from build123d import *

# Parameters (mm, degrees)
SKETCH2_W           = 15
SKETCH2_H           = 20
SKETCH2_W_2         = 23
SKETCH2_H_2         = 15
BOSS_EXTRUDE1_DEPTH = 10


with BuildPart() as part:
    # Sketch2 → Boss-Extrude1 (new body)
    with BuildSketch(Plane.XY):
        Polygon((0, 0), (120, 0), (120, 10), (180, 10), (180, 0), (240, 0), (240, 10), (300, 10), (300, 0), (420, 0), (420, -75), (430, -75), (430, -120), (420, -120), (420, -165), (430, -165), (430, -210), (420, -210), (420, -285), (300, -285), (300, -295), (240, -295), (240, -285), (180, -285), (180, -295), (120, -295), (120, -285), (0, -285), (0, -210), (-10, -210), (-10, -165), (0, -165), (0, -120), (-10, -120), (-10, -75), (0, -75), align=None)
        with Locations((144.916665259, -151.561421388)):
            Rectangle(SKETCH2_W, SKETCH2_H, mode=Mode.SUBTRACT)
        with Locations((338.315226992, -153.118682745)):
            Rectangle(SKETCH2_W, SKETCH2_H, mode=Mode.SUBTRACT)
        with Locations((376.315226992, -153.118682745)):
            Rectangle(SKETCH2_W, SKETCH2_H, mode=Mode.SUBTRACT)
        with Locations((338.315226992, -239.118682745)):
            Rectangle(SKETCH2_W, SKETCH2_H, mode=Mode.SUBTRACT)
        with Locations((44.5, -152)):
            Rectangle(SKETCH2_W, SKETCH2_H, mode=Mode.SUBTRACT)
        with Locations((82.5, -152)):
            Rectangle(SKETCH2_W, SKETCH2_H, mode=Mode.SUBTRACT)
        with Locations((44.5, -238)):
            Rectangle(SKETCH2_W, SKETCH2_H, mode=Mode.SUBTRACT)
        with Locations((82.5, -238)):
            Rectangle(SKETCH2_W, SKETCH2_H, mode=Mode.SUBTRACT)
        with Locations((63.5, -193.5)):
            Rectangle(SKETCH2_W_2, SKETCH2_H_2, mode=Mode.SUBTRACT)
        with Locations((182.916665259, -151.561421388)):
            Rectangle(SKETCH2_W, SKETCH2_H, mode=Mode.SUBTRACT)
        with Locations((144.916665259, -237.561421388)):
            Rectangle(SKETCH2_W, SKETCH2_H, mode=Mode.SUBTRACT)
        with Locations((182.916665259, -237.561421388)):
            Rectangle(SKETCH2_W, SKETCH2_H, mode=Mode.SUBTRACT)
        with Locations((163.916665259, -193.061421388)):
            Rectangle(SKETCH2_W_2, SKETCH2_H_2, mode=Mode.SUBTRACT)
        with Locations((242.869049507, -152.216184795)):
            Rectangle(SKETCH2_W, SKETCH2_H, mode=Mode.SUBTRACT)
        with Locations((280.869049507, -152.216184795)):
            Rectangle(SKETCH2_W, SKETCH2_H, mode=Mode.SUBTRACT)
        with Locations((242.869049507, -238.216184795)):
            Rectangle(SKETCH2_W, SKETCH2_H, mode=Mode.SUBTRACT)
        with Locations((280.869049507, -238.216184795)):
            Rectangle(SKETCH2_W, SKETCH2_H, mode=Mode.SUBTRACT)
        with Locations((261.869049507, -193.716184795)):
            Rectangle(SKETCH2_W_2, SKETCH2_H_2, mode=Mode.SUBTRACT)
        with Locations((376.315226992, -239.118682745)):
            Rectangle(SKETCH2_W, SKETCH2_H, mode=Mode.SUBTRACT)
        with Locations((357.315226992, -194.618682745)):
            Rectangle(SKETCH2_W_2, SKETCH2_H_2, mode=Mode.SUBTRACT)
    extrude(amount=BOSS_EXTRUDE1_DEPTH)


solid = part.part
Verification items for the finished model (mm, model axes). A direction names the side the tool comes from. Give positions to 0.01 mm unless a question says otherwise; leave off trailing zeros. Write each loop counter-clockwise with the first axis right and the second up, starting at its lowest first coordinate (ties: lowest second). Pieces come first, ordered by that corner, then holes. Notation, with made-up numbers: M -9.75,9.25 L -0.75,9.25 A24 ccw -0.75,41.25 Z; hole C -31,42.5 d1. An arc over 180 degrees is marked long. Use CSV: the item, a comma, the result in double quotes.
1) Material ranges on line 1 along Y through (x, z) = (185.5, 4.25); line 2 along Y through (x, z) = (281.5, 1.25); line 3 along Y through (x, z) = (171, 9.25), recorded low to high.
Final values:
line 1,"-285 to -247.56, -227.56 to -161.56, -141.56 to 0"
line 2,"-295 to -248.22, -228.22 to -162.22, -142.22 to 10"
line 3,"-295 to -200.56, -185.56 to 10"
2) Access from +Z, -Z, +X, -X, +Y, -Y to the whole of each face (thin tool, end or side, straight path). Record for faces 1 (the face through (425, -165, 5)), 2 (the face through (-5, -210, 5)), 3 (the face through (425, -75, 5)), 4 (the face through (240, 5, 5)), 5 (the face through (338, -229.119, 5)).
Final values:
face 1,"+Z, -Z, +X"
face 2,"+Z, -Z, -X, -Y"
face 3,"+Z, -Z, +X, +Y"
face 4,"+Z, -Z, +Y"
face 5,"+Z, -Z"
3) Go/stop test with flat-tipped pins: pin 1 Ø3 at (y, z) = (-288, 7) entering from +X; pin 2 Ø3 at (x, z) = (373.5, 4) entering from +Y; pin 3 Ø3 at (x, z) = (360.5, 5) entering from -Y. Record where each tip stops, or that it passes through.
Final values:
pin 1,"x = 300"
pin 2,"y = 0"
pin 3,"y = -285"
4) Release check for a two-part mould opening along Y. For faces 6 (the face through (61, -285, 5)), 7 (the face through (75, -152, 5)), 8 (the face through (-10, -98, 5)) record: released by +Y, released by -Y, zero draft, split by the parting line, or undercut.
Final values:
face 6,"released by -Y"
face 7,"undercut"
face 8,"zero draft"
5) Cross-section at A-A (y = -151). State how many separate pieces and enclosed holes the cut face has, plus the area to 3 significant figures.
Final values:
separate pieces,"9"
enclosed holes,"0"
area,"3,000 mm²"
6) Cross-section at C-C (x = 207). Enter the section's corners in (y, z).
Final values:
outline,"M -285,0 L 0,0 L 0,10 L -285,10 Z"
